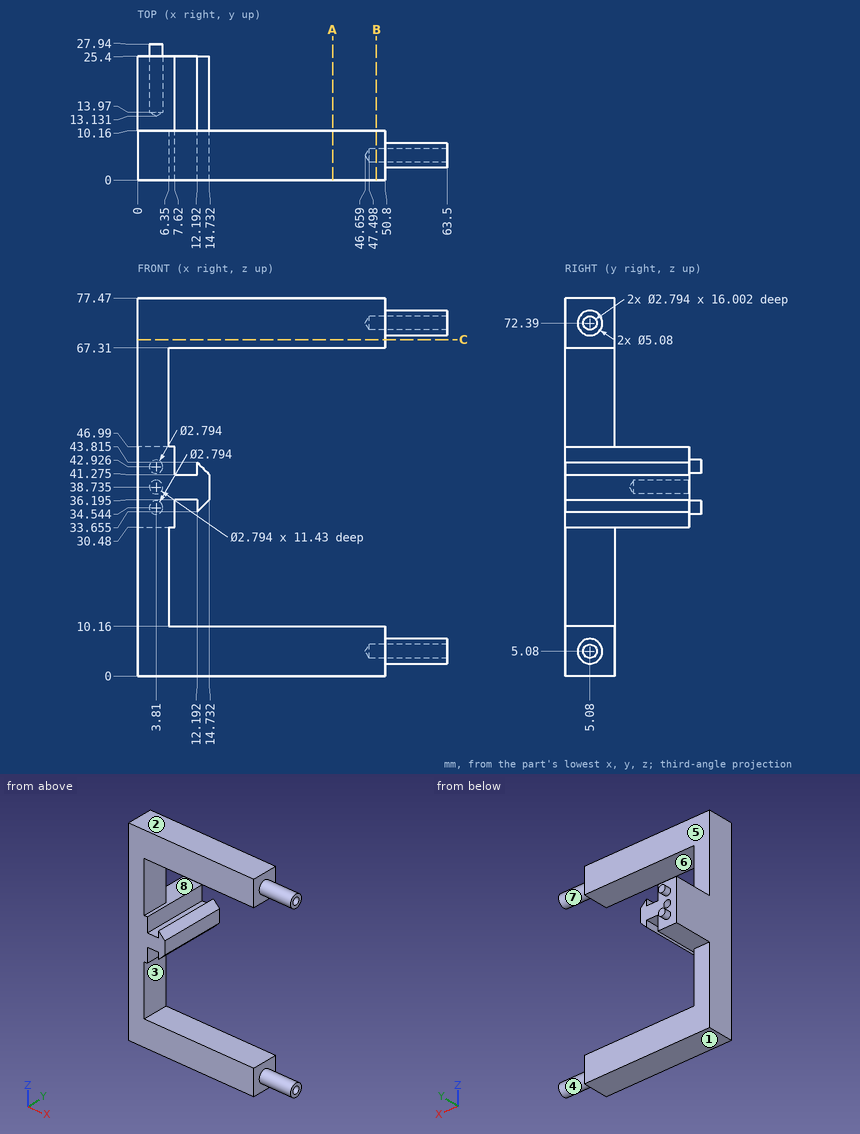
Design review of the part shown in the three views and the two pictorial views. Dimensions are in mm from the part's minimum x, y and z. A direction names the side the tool comes from. Round coordinates to 2 decimals unless told otherwise and drop trailing zeros. Write each loop counter-clockwise with the first axis right and the second up, starting at its lowest first coordinate (ties: lowest second). Pieces come first, ordered by that corner, then holes. Notation, with made-up numbers: (-6, 82) - (16, 82) arc R6 ccw to (16, 86) - close; hole circle Ø7 at (-40, -16). An arc over 180 degrees is marked (long way). Return JSON: item names as keys, results as strings. Group by question number.
Item 1: We need section A-A on x = 40. Write out the cut boundary in (y, z).
Item 2: We need section C-C on z = 69. Write out the cut boundary in (x, y), and give its area (3 significant figures).
Item 3: For probe 1 along Z at (x, y) = (3.81, 21.25); probe 2 along Y at (x, z) = (54.75, 5.08); probe 3 along Z at (x, y) = (16, 9.75), list the stretches that pass through material, from the lowest coordinate up. Write a range as [from, to].
Item 4: The part is to be moulded in two halves that separate along Z. For the marked faces 1, 2, 3 and 4, say which applies: pulls with the +Z half, pulls with the -Z half, needs draft (parallel to the pull), parting line crosses it, or undercut.
Item 5: We need section B-B on x = 49. Write out the cut boundary in (y, z), and give its area (3 significant figures).
Item 6: Machinability: for the marked faces 5, 6, 7 and 8, which of the approach directions +Z, -Z, +X, -X, +Y, -Y give a long, thin tool a straight path to every point of the face, cutting with its end or side? Answer none if there is none.
Item 7: Insertion check: P1, Ø2.5, axis at y = 5.08, z = 72.39, coming from the -X side; P2, Ø8, axis at y = 7, z = 52.5, coming from the +X side; P3, Ø5.5, axis at y = 16, z = 39, coming from the +X side; P4, Ø2.5, axis at x = 11, y = 16.5, coming from the +Z side (3 decimals). Each pin has a flat end and moves straight along its axis. Give the tip position at first contact, or say it passes through.
Model answer:
{
 "1": {"outline": "(0, 0) - (10.16, 0) - (10.16, 10.16) - (0, 10.16) - close; (0, 67.31) - (10.16, 67.31) - (10.16, 77.47) - (0, 77.47) - close"},
 "2": {"outline": "(0, 0) - (50.8, 0) - (50.8, 10.16) - (0, 10.16) - close", "area": "516 mm²"},
 "3": {"probe 1": "z = [30.48, 37.34], [40.13, 46.99]", "probe 2": "y = [2.54, 3.68], [6.48, 7.62]", "probe 3": "z = [0, 10.16], [67.31, 77.47]"},
 "4": {"face 1": "pulls with the -Z half", "face 2": "pulls with the +Z half", "face 3": "undercut", "face 4": "undercut"},
 "5": {"outline": "(0, 0) - (10.16, 0) - (10.16, 10.16) - (0, 10.16) - close; (0, 67.31) - (10.16, 67.31) - (10.16, 77.47) - (0, 77.47) - close; hole circle Ø2.79 at (5.08, 5.08); hole circle Ø2.79 at (5.08, 72.39)", "area": "194 mm²"},
 "6": {"face 5": "+Z, +X, -X, +Y", "face 6": "+X, +Y, -Y", "face 7": "+X", "face 8": "+X, +Y"},
 "7": {"P1": "stops at x = 0", "P2": "stops at x = 6.35", "P3": "stops at x = 14.73", "P4": "stops at z = 43.815"}
}
